Study the drawing (mm; zero at the part's minimum x, y, z) and answer. Round coordinates to 2 decimals unless told otherwise and drop trailing zeros. Write each loop counter-clockwise with the first axis right and the second up, starting at its lowest first coordinate (ties: lowest second). Pieces come first, ordered by that corner, then holes. Notation, with made-up numbers: (2.25, -16.5) - (37.25, -16.5) arc R14 ccw to (37.25, 0.5) - close; hole circle Ø6 at (47.5, 20). An arc over 180 degrees is marked (long way). Return JSON: item names as keys, results as strings. Group by question number.
(1) Each of these flat-tipped pins is pushed along its axis until it touches: pin 1 (2 mm diameter, centred on y = 438, z = 6, fed in from +X); pin 2 (5 mm diameter, centred on y = 235, z = 10, fed in from -X) (3 decimals); pin 3 (4 mm diameter, centred on x = 95, z = 6.5, fed in from +Y); pin 4 (8 mm diameter, centred on x = 74, y = 119, fed in from -Z). Where does it stop, or does it pass through?
(2) Section C-C, the plane y = 585.5 is taken. Write down the section's boundary in (x, z), then the cut area to 3 significant figures.
(3) Section A-A, the plane z = 8.5 is taken. Write down the section's boundary in (x, y), then the cut area to 3 significant figures.
(4) Find the intervals of material crossed by line 1 along Y through (x, z) = (56, 11.5); line 2 along Y through (x, z) = (65, 7); line 3 along Y through (x, z) = (108, 7.5), in increasing order. Write a range as [from, to].
(5) Section B-B, the plane y = 288.5 is taken. Write down the section's boundary in (x, z).
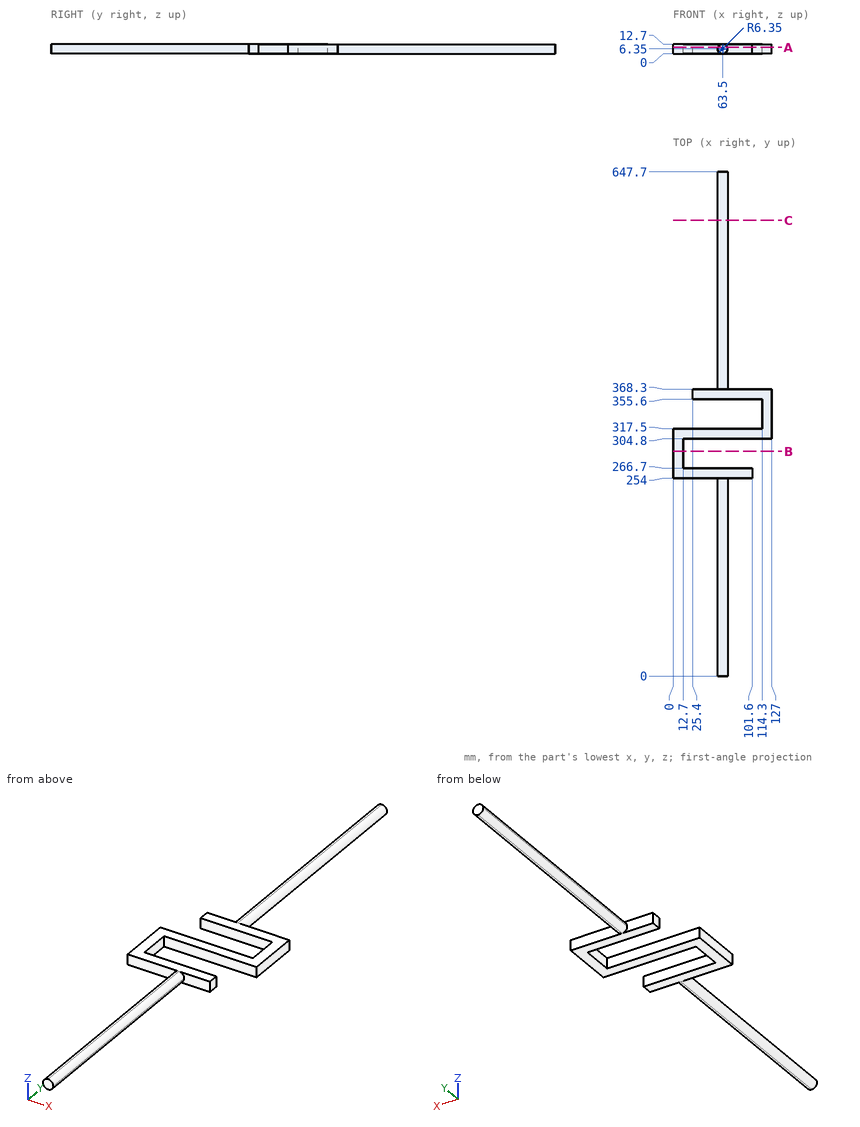
Working result:
{
 "1": {"pin 1": "stops at x = 69.85", "pin 2": "stops at x = 57.255", "pin 3": "stops at y = 368.3", "pin 4": "passes through"},
 "2": {"outline": "circle Ø12.7 at (63.5, 6.35)", "area": "127 mm^2"},
 "3": {"outline": "(0, 254) - (57.53, 254) - (57.53, 0) - (69.47, 0) - (69.47, 254) - (101.6, 254) - (101.6, 266.7) - (12.7, 266.7) - (12.7, 304.8) - (127, 304.8) - (127, 368.3) - (69.47, 368.3) - (69.47, 647.7) - (57.53, 647.7) - (57.53, 368.3) - (25.4, 368.3) - (25.4, 355.6) - (114.3, 355.6) - (114.3, 317.5) - (0, 317.5) - close", "area": "11,500 mm^2"},
 "4": {"line 1": "y = [254, 266.7], [304.8, 317.5], [355.6, 368.3]", "line 2": "y = [0, 266.7], [304.8, 317.5], [355.6, 647.7]", "line 3": "y = [304.8, 317.5], [355.6, 368.3]"},
 "5": {"outline": "(0, 0) - (12.7, 0) - (12.7, 12.7) - (0, 12.7) - close"}
}
